Here's how the part is built. I have some questions about the finished solid (model axes, mm). A direction names the side the tool comes from. Round coordinates to 2 decimals unless told otherwise and drop trailing zeros. Order: outer loops, then holes, each group sorted by start corner. A loop starts at its lowest first (then second) coordinate and runs counter-clockwise, first axis right, second up. Notation, with made-up numbers: (20.5, -4.5) -> (24.5, -4.5) arc R18 ccw to (24.5, 6.5) -> close; hole circle Ø4 at (57, 76). An arc over 180 degrees is marked (long way). Use a Markdown table: item, result. Add a question column.
(1) On a 3-axis mill with a long thin cutter (end or side, diameter ignored), from which of +Z, -Z, +X, -X, +Y, -Y can I reach the whole of each face in a straight line? I mean faces 4 (the face through (50, 0, 0)), 5 (the face through (-10, -124, 0)), 6 (the face through (301.923, -166.245, 0.245)), 7 (the face through (-1, -25, 0)), 8 (the face through (66, -151, -22.5)). Say none if no direction works.
(2) I want a section at C-C, the plane x = 290. Please give me the cut outline in (y, z), then the cut area to 3 significant figures.
(3) I want a section at B-B, the plane z = -0.5. Please give me the cut outline in (x, y), then the cut area to 3 significant figures.
(4) If I drill on probe 1 along Y at (x, z) = (6, 13); probe 2 along Y at (x, z) = (290, 19); probe 3 along Y at (x, z) = (68, 12.5), over which ranges is the centre line in solid material (lowest first)?
(5) I want a section at D-D, the plane y = -123. Please give me the cut outline in (x, z), then the cut area to 3 significant figures.
(6) Thinking about a two-plate mould opening in Y: for faces 1 (the face through (-1, 25, 0)), 2 (the face through (0, -70, 0)), 3 (the face through (260, -170, 0)), which applies, pulls with the +Y half, pulls with the -Y half, needs draft (parallel to the pull), parting line crosses it, or undercut?
(7) I'm going to push flat-ended pins straight in: P1, Ø17.5, axis at y = 6.5, z = 7.5, coming from the +X side; P2, Ø6, axis at x = 290, y = -170, coming from the -Z side; P3, Ø5.5, axis at y = -1.5, z = -19.5, coming from the +X side; P4, Ø10.5, axis at x = -2, z = -1.5, coming from the -Y side. Where does each tip first touch, or does it pass through?
(8) I want a section at A-A, the plane y = -170. Please give me the cut outline in (x, z), then the cut area to 3 significant figures.
from build123d import *

# Parameters (mm, degrees)
SKETCH1_W           = 100
SKETCH1_H           = 50
BOSS_EXTRUDE1_DEPTH = 17.5
SKETCH2_R           = 5
BOSS_EXTRUDE2_DEPTH = 5
BOSS_EXTRUDE3_DEPTH = 17.5
FILLET1_R           = 15
SKETCH5_R           = 12.5
SKETCH5_R_2         = 5
BOSS_EXTRUDE4_DEPTH = 17.5


with BuildPart() as part:
    # Sketch1 → Boss-Extrude1 (new, symmetric)
    with BuildSketch(Plane.XY):
        Rectangle(SKETCH1_W, SKETCH1_H)
    extrude(amount=BOSS_EXTRUDE1_DEPTH, both=True)

    # Sketch2 → Boss-Extrude2 (add)
    with BuildSketch(Plane.XY.offset(17.5)):
        Polygon((20, -40), (65, -40), (65, 40), (-65, 40), (-65, -40), (-20, -40), (-20, -190), (20, -190), (270, -190), (310, -190), (310, -150), (270, -150), (20, -150), align=None)
        with Locations((290, -170)):
            Circle(SKETCH2_R, mode=Mode.SUBTRACT)
    boss_extrude2 = extrude(amount=BOSS_EXTRUDE2_DEPTH)

    # Mirror1: Boss-Extrude2 across plane
    add(boss_extrude2.mirror(Plane.XY))

    # Sketch4 → Boss-Extrude3 (add, symmetric)
    with BuildSketch(Plane.XY):
        Polygon((-10, -70), (-10, -180), (260, -180), (260, -160), (10, -160), (10, -70), align=None)
    extrude(amount=BOSS_EXTRUDE3_DEPTH, both=True)

    # Fillet1
    fillet1_edges = [part.edges().sort_by_distance(p)[0] for p in [
        (310, -190, 20),
        (310, -150, 20),
        (310, -150, -20),
        (310, -190, -20),
    ]]
    fillet(fillet1_edges, radius=FILLET1_R)

    # Sketch5 → Boss-Extrude4 (add, symmetric)
    with BuildSketch(Plane.XY):
        with Locations((290, -170)):
            Circle(SKETCH5_R)
        with Locations((290, -170)):
            Circle(SKETCH5_R_2, mode=Mode.SUBTRACT)
    extrude(amount=BOSS_EXTRUDE4_DEPTH, both=True)


solid = part.part
Taken from the geometry:
| question | item | result |
|---|---|---|
| 1 | face 4 | +X, +Y |
| 1 | face 5 | -X, -Y |
| 1 | face 6 | none |
| 1 | face 7 | +X, -X |
| 1 | face 8 | -Z, +X, -X, +Y, -Y |
| 2 | outline | (-190, -22.5) -> (-175, -22.5) -> (-175, 22.5) -> (-190, 22.5) -> (-190, 17.5) -> (-182.5, 17.5) -> (-182.5, -17.5) -> (-190, -17.5) -> close; (-165, -22.5) -> (-150, -22.5) -> (-150, -17.5) -> (-157.5, -17.5) -> (-157.5, 17.5) -> (-150, 17.5) -> (-150, 22.5) -> (-165, 22.5) -> close |
| 2 | area | 825 mm2 |
| 3 | outline | (-50, -25) -> (50, -25) -> (50, 25) -> (-50, 25) -> close; (-10, -180) -> (260, -180) -> (260, -160) -> (10, -160) -> (10, -70) -> (-10, -70) -> close; circle Ø25 at (290, -170); hole circle Ø10 at (290, -170) |
| 3 | area | 12,600 mm2 |
| 4 | probe 1 | y = -180 to -70, -25 to 25 |
| 4 | probe 2 | y = -190 to -175, -165 to -150 |
| 4 | probe 3 | y = -180 to -160 |
| 5 | outline | (-20, -22.5) -> (20, -22.5) -> (20, -17.5) -> (10, -17.5) -> (10, 17.5) -> (20, 17.5) -> (20, 22.5) -> (-20, 22.5) -> (-20, 17.5) -> (-10, 17.5) -> (-10, -17.5) -> (-20, -17.5) -> close |
| 5 | area | 1,100 mm2 |
| 6 | face 1 | pulls with the +Y half |
| 6 | face 2 | undercut |
| 6 | face 3 | needs draft |
| 7 | P1 | stops at x = 50 |
| 7 | P2 | passes through |
| 7 | P3 | stops at x = 65 |
| 7 | P4 | stops at y = -180 |
| 8 | outline | (-20, -22.5) -> (285, -22.5) -> (285, 22.5) -> (-20, 22.5) -> (-20, 17.5) -> (-10, 17.5) -> (-10, -17.5) -> (-20, -17.5) -> close; (295, -22.5) -> (310, -22.5) -> (310, -17.5) -> (302.5, -17.5) -> (302.5, 17.5) -> (310, 17.5) -> (310, 22.5) -> (295, 22.5) -> close; hole (260, -17.5) -> (277.5, -17.5) -> (277.5, 17.5) -> (260, 17.5) -> close |
| 8 | area | 13,200 mm2 |
